Check sheet for the modelled part. Datum: model origin and axes. Units: mm. Give positions to 0.01 mm unless a question says otherwise; leave off trailing zeros.
```python
from build123d import *

# Parameters (mm, degrees)
F0_W     = 110
F0_H     = 40
F1_DEPTH = 25
F2_W     = 3
F2_H     = 25
F3_DEPTH = 20
F4_R     = 0.9


with BuildPart() as f1:
    # F0 (on Top) → F1 (new body)
    with BuildSketch(Plane.XY):
        with Locations((0.478346, 3.515624)):
            Rectangle(F0_W, F0_H)
    extrude(amount=F1_DEPTH)

    # F2 (on face) → F3 (cut)
    with BuildSketch(Plane.XY.offset(25)):
        with Locations((-45.382225, 4.651876)):
            Rectangle(F2_W, F2_H)
        Polygon((-36.882324, 17.171759), (-36.882324, -7.828241), (-33.882324, -7.828241), (-33.882324, 17.01556), align=None)
        Polygon((-26.882324, 17.171759), (-26.882324, -7.828241), (-23.882324, -7.828241), (-23.882324, 17.01556), align=None)
        Polygon((-16.882324, 17.171759), (-16.882324, -7.828241), (-13.882324, -7.828241), (-13.882324, 17.01556), align=None)
        Polygon((-6.882324, 17.171759), (-6.882324, -7.828241), (-3.882324, -7.828241), (-3.882324, 17.01556), align=None)
        Polygon((3.117676, 17.171759), (3.117676, -7.828241), (6.117676, -7.828241), (6.117676, 17.01556), align=None)
        Polygon((13.117676, 17.171759), (13.117676, -7.828241), (16.117676, -7.828241), (16.117676, 17.01556), align=None)
        Polygon((23.117676, 17.171759), (23.117676, -7.828241), (26.117676, -7.828241), (26.117676, 17.01556), align=None)
        Polygon((33.117676, 17.171759), (33.117676, -7.828241), (36.117676, -7.828241), (36.117676, 17.01556), align=None)
        Polygon((43.117676, 17.171759), (43.117676, -7.828241), (46.117676, -7.828241), (46.117676, 17.01556), align=None)
    extrude(amount=-F3_DEPTH, mode=Mode.SUBTRACT)

    # F4
    f4_edges = [f1.edges().sort_by_distance(p)[0] for p in [
        (0.478346, -16.484376, 25),
        (-54.521654, 3.515624, 25),
        (55.478346, 3.515624, 25),
        (0.478346, 23.515624, 25),
        (-46.882225, 4.651876, 25),
        (-45.382225, -7.848124, 25),
        (-43.882225, 4.651876, 25),
        (-45.382225, 17.151876, 25),
        (-36.882324, 4.671759, 25),
        (-35.382324, -7.828241, 25),
        (-33.882324, 4.593659, 25),
        (-35.382324, 17.093659, 25),
        (-26.882324, 4.671759, 25),
        (-25.382324, -7.828241, 25),
        (-23.882324, 4.593659, 25),
        (-25.382324, 17.093659, 25),
        (-16.882324, 4.671759, 25),
        (-15.382324, -7.828241, 25),
        (-13.882324, 4.593659, 25),
        (-15.382324, 17.093659, 25),
        (-6.882324, 4.671759, 25),
        (-5.382324, -7.828241, 25),
        (-3.882324, 4.593659, 25),
        (-5.382324, 17.093659, 25),
        (3.117676, 4.671759, 25),
        (4.617676, -7.828241, 25),
        (6.117676, 4.593659, 25),
        (4.617676, 17.093659, 25),
        (13.117676, 4.671759, 25),
        (14.617676, -7.828241, 25),
        (16.117676, 4.593659, 25),
        (14.617676, 17.093659, 25),
        (23.117676, 4.671759, 25),
        (24.617676, -7.828241, 25),
        (26.117676, 4.593659, 25),
        (24.617676, 17.093659, 25),
        (33.117676, 4.671759, 25),
        (34.617676, -7.828241, 25),
        (36.117676, 4.593659, 25),
        (34.617676, 17.093659, 25),
        (43.117676, 4.671759, 25),
        (44.617676, -7.828241, 25),
        (46.117676, 4.593659, 25),
        (44.617676, 17.093659, 25),
    ]]
    fillet(f4_edges, radius=F4_R)


solid = f1.part
```
(1) Gauge pin test, flat ends, axial feed: pin 1 Ø3.5 at (x, y) = (34.5, -0.5) entering from +Z; pin 2 Ø1.5 at (x, y) = (4, 9) entering from +Z. Record the tip position at first contact, or that the pin passes through.
Response values:
pin 1: stops at z = 24.83
pin 2: stops at z = 5
(2) Cross-section at A-A on z = 6. Count the separate pieces of the cut face and the enclosed holes in it, then the cut area to 3 significant figures.
Response values:
separate pieces: 1
enclosed holes: 10
area: 3,650 mm2
(3) Material ranges on L1, parallel to Z at x = 25, y = -2; L2, parallel to Y at x = -16, z = 10.5; L3, parallel to Z at x = 45, y = -8, recorded low to high.
Response values:
L1: z = 0 to 5
L2: y = -16.48 to -7.83, 17.13 to 23.52
L3: z = 0 to 24.63
(4) Release check for a two-part mould opening along X. For faces 1 (the face through (0, 4, 0)), 2 (the face through (-13.882, 4, 15)) record: released by +X, released by -X, zero draft, split by the parting line, or undercut.
Response values:
face 1: zero draft
face 2: undercut
